Design review of the part built by this model. Coordinates are the model's own, in mm. Face numbers are marked on the shaded views. A direction names the side the tool comes from. Coordinates: 2 decimals unless noted, no trailing zeros. Order: outer loops, then holes, each group sorted by start corner. A loop starts at its lowest first (then second) coordinate and runs counter-clockwise, first axis right, second up. Notation, with made-up numbers: M -29.75,51 L -24.75,51 A20 ccw -24.75,58 Z; hole C -22,-35.5 d5. An arc over 180 degrees is marked long. Use CSV: the item, a comma, the result in double quotes.
```python
from build123d import *

# Parameters (mm, degrees)
F0_W     = 248.435066
F0_H     = 182.613314
F0_W_2   = 226.806744
F0_H_2   = 155.059486
F1_DEPTH = 100
F2_W     = 75.79172
F2_H     = 48.828578
F3_DEPTH = 182.614313
F4_R     = 12.665066
F5_DEPTH = 248.436065


with BuildPart() as f1:
    # F0 (on Top) → F1 (new body)
    with BuildSketch(Plane.XY):
        Rectangle(F0_W, F0_H)
        Rectangle(F0_W_2, F0_H_2, mode=Mode.SUBTRACT)
    extrude(amount=F1_DEPTH)

    # F2 (on face) → F3 (cut, through all)
    with BuildSketch(Plane.XZ.offset(91.306657)):
        with Locations((0.759939, 75.585711)):
            Rectangle(F2_W, F2_H)
    extrude(amount=-F3_DEPTH, mode=Mode.SUBTRACT)

    # F4 (on face) → F5 (cut, through all)
    with BuildSketch(Plane.YZ.offset(124.217533)):
        with Locations((0, 36.991738)):
            Circle(F4_R)
    extrude(amount=-F5_DEPTH, mode=Mode.SUBTRACT)


solid = f1.part
```
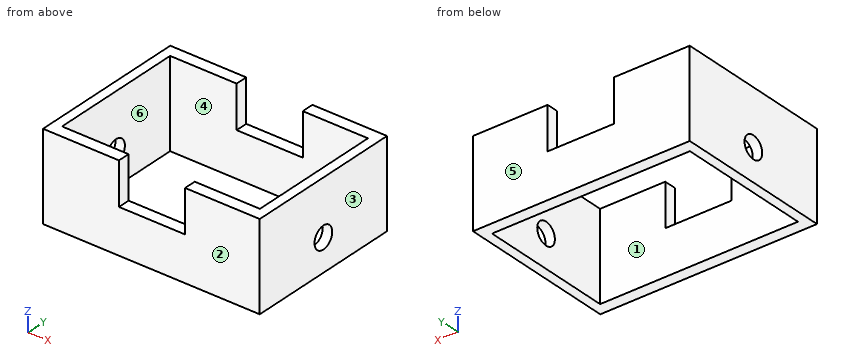
(1) Add section C-C on y = 0. State the section outline as (x, z) points, and give its area (3 significant figures).
The answers:
outline,"M -124.22,0 L -113.4,0 L -113.4,24.33 L -124.22,24.33 Z; M -124.22,49.66 L -113.4,49.66 L -113.4,100 L -124.22,100 Z; M 113.4,0 L 124.22,0 L 124.22,24.33 L 113.4,24.33 Z; M 113.4,49.66 L 124.22,49.66 L 124.22,100 L 113.4,100 Z"
area,"1,610 mm2"
(2) Add section D-D on z = 74. State the section outline as (x, y) points.
The answers:
outline,"M -124.22,-91.31 L -37.14,-91.31 L -37.14,-77.53 L -113.4,-77.53 L -113.4,77.53 L -37.14,77.53 L -37.14,91.31 L -124.22,91.31 Z; M 38.66,-91.31 L 124.22,-91.31 L 124.22,91.31 L 38.66,91.31 L 38.66,77.53 L 113.4,77.53 L 113.4,-77.53 L 38.66,-77.53 Z"
(3) Wall thickness on probe 1 along Z at (x, y) = (117.75, 0); probe 2 along Y at (x, z) = (-43, 69); probe 3 along X at (y, z) = (41, 90): over which ranges is each line inside the solid? List them lowest first.
The answers:
probe 1,"z = 0 to 24.33, 49.66 to 100"
probe 2,"y = -91.31 to -77.53, 77.53 to 91.31"
probe 3,"x = -124.22 to -113.4, 113.4 to 124.22"
(4) Clearance check with flat-ended pins moving along their axes: P1, Ø23, axis at y = 0, z = 36.99, coming from the -X side; P2, Ø11, axis at x = -16.5, y = -86.5, coming from the +Z side. State where each tip first meets the part, or that it passes through.
The answers:
P1,"passes through"
P2,"stops at z = 51.17"
(5) The part is to be moulded in two halves that separate along Y. For the marked faces 1, 2, 3 and 4, say which applies: pulls with the +Y half, pulls with the -Y half, needs draft (parallel to the pull), parting line crosses it, or undercut.
The answers:
face 1,"undercut"
face 2,"pulls with the -Y half"
face 3,"needs draft"
face 4,"undercut"
(6) Add section B-B on y = -71.5. State the section outline as (x, z) points.
The answers:
outline,"M -124.22,0 L -113.4,0 L -113.4,100 L -124.22,100 Z; M 113.4,0 L 124.22,0 L 124.22,100 L 113.4,100 Z"
(7) For the marked faces 5 and 6, list the 3-axis set-ups (+Z, -Z, +X, -X, +Y, -Y) from which the entire face can be reached by the end or side of a thin tool; tool diameter is ignored.
The answers:
face 5,"+Z, -Z, +X, -X, +Y"
face 6,"+Z, -Z"
(8) Add section A-A on x = 10. State the section outline as (y, z) points.
The answers:
outline,"M -91.31,0 L -77.53,0 L -77.53,51.17 L -91.31,51.17 Z; M 77.53,0 L 91.31,0 L 91.31,51.17 L 77.53,51.17 Z"
